Geometry check sheet. Reference: the model listing, model coordinates, mm. Face numbers are marked on the shaded views. A direction names the side the tool comes from. Give positions to 0.01 mm unless a question says otherwise; leave off trailing zeros. Write each loop counter-clockwise with the first axis right and the second up, starting at its lowest first coordinate (ties: lowest second). Pieces come first, ordered by that corner, then holes.
(1) Cross-section at C-C (z = -8). Record the boundary of the cut face in (x, y), and give its area (3 significant figures).
(2) Cross-section at B-B (y = 13.25). Record the boundary of the cut face in (x, z).
(3) Cross-section at A-A (z = 3). Record the boundary of the cut face in (x, y).
(4) Tool access check on the marked faces 4, 5, 6 and 7. Record the directions out of +Z, -Z, +X, -X, +Y, -Y that give a thin tool (end or side, any length) a straight path to the whole face; none if there is none.
(5) Mould release check, pull along Z, two halves, no side actions. Record for the marked faces 1, 2 and 3: +Z half, -Z half, draft (parallel to the pull), parting line (faces both ways), or undercut.
(6) Thickness scan on line 1 along Z through (x, y) = (-8.75, 5); line 2 along X through (y, z) = (10, -0.5); line 3 along Y through (x, z) = (22, 3.65). Record the ranges inside material, lowest first.
(7) Cross-section at D-D (x = 15). Record the boundary of the cut face in (y, z), and give its area (3 significant figures).
(8) Depth check by flat-ended pin: P1, Ø5, axis at x = -9, y = 8, coming from the -Z side; P2, Ø5, axis at x = 13.5, z = -1.5, coming from the -Y side; P3, Ø3, axis at x = 22, y = 9.5, coming from the -Z side; P4, Ø8, axis at x = 13.5, y = 13, coming from the +Z side. Enter the tip coordinate at first touch or a pass-through.
```python
from build123d import *

# Parameters (mm, degrees)
SKETCH1_W           = 50
SKETCH1_H           = 36
BOSS_EXTRUDE1_DEPTH = 3
SKETCH2_W           = 5
SKETCH2_H           = 8
SKETCH2_W_2         = 6
SKETCH2_H_2         = 20
BOSS_EXTRUDE2_DEPTH = 14
SKETCH3_W           = 15
SKETCH3_H           = 4
BOSS_EXTRUDE3_DEPTH = 13
SKETCH4_R           = 3
BOSS_EXTRUDE4_DEPTH = 2
SKETCH5_R           = 2
CUT_EXTRUDE1_DEPTH  = 12
CUT_EXTRUDE2_DEPTH  = 11
SKETCH7_W           = 1.666666666
SKETCH7_H           = 10
BOSS_EXTRUDE5_DEPTH = 14
CUT_EXTRUDE3_REACH  = 45.218
CUT_EXTRUDE4_REACH  = 36.943
SKETCH10_W          = 10
SKETCH10_H          = 1.666666667
BOSS_EXTRUDE7_DEPTH = 13
CUT_EXTRUDE5_DEPTH  = 2
SKETCH12_R          = 2
CUT_EXTRUDE6_DEPTH  = 6
CHAMFER1_SIZE       = 2
CHAMFER1_SIZE2      = 4
CUT_EXTRUDE7_DEPTH  = 5
SKETCH14_R          = 1.3
CUT_EXTRUDE8_DEPTH  = 6
SKETCH15_R          = 1
CUT_EXTRUDE9_DEPTH  = 6


with BuildPart() as part:
    # Sketch1 → Boss-Extrude1 (new body)
    with BuildSketch(Plane(origin=(0, 0, 0), x_dir=(1, 0, 0), z_dir=(0, 1, 0))):
        Rectangle(SKETCH1_W, SKETCH1_H)
    extrude(amount=BOSS_EXTRUDE1_DEPTH)

    # Sketch2 → Boss-Extrude2 (add)
    with BuildSketch(Plane(origin=(0, 3, 0), x_dir=(1, 0, 0), z_dir=(0, 1, 0))):
        with Locations((22.5, -4)):
            Rectangle(SKETCH2_W, SKETCH2_H)
        with Locations((-8, 2)):
            Rectangle(SKETCH2_W_2, SKETCH2_H_2)
    extrude(amount=BOSS_EXTRUDE2_DEPTH)

    # Sketch3 → Boss-Extrude3 (add)
    with BuildSketch(Plane(origin=(0, 3, 0), x_dir=(1, 0, 0), z_dir=(0, 1, 0))):
        with Locations((10, 16)):
            Rectangle(SKETCH3_W, SKETCH3_H)
    extrude(amount=BOSS_EXTRUDE3_DEPTH)

    # Sketch4 → Boss-Extrude4 (add)
    with BuildSketch(Plane(origin=(0, 0, -18), x_dir=(-1, 0, 0), z_dir=(0, 0, -1))):
        with Locations(Location((-13.5, 9.25, 0), (0, 0, 180))):
            Circle(SKETCH4_R)
    extrude(amount=BOSS_EXTRUDE4_DEPTH)

    # Sketch5 → Cut-Extrude1 (cut)
    with BuildSketch(Plane(origin=(0, 0, -20), x_dir=(-1, 0, 0), z_dir=(0, 0, -1))):
        with Locations((-13.5, 9.25)):
            Circle(SKETCH5_R)
    extrude(amount=-CUT_EXTRUDE1_DEPTH, mode=Mode.SUBTRACT)

    # Sketch6 → Cut-Extrude2 (cut)
    with BuildSketch(Plane(origin=(0, 3, 0), x_dir=(1, 0, 0), z_dir=(0, 1, 0))):
        Polygon((-11, 12), (-11, 18), (-25, 18), (-25, -18), (25, -18), (25, -8), (-11, -8), align=None)
    extrude(amount=-CUT_EXTRUDE2_DEPTH, mode=Mode.SUBTRACT)

    # Sketch7 → Boss-Extrude5 (add)
    with BuildSketch(Plane(origin=(0, 17, 0), x_dir=(1, 0, 0), z_dir=(0, 1, 0))):
        with Locations((22.5, 5)):
            Rectangle(SKETCH7_W, SKETCH7_H)
    extrude(amount=-BOSS_EXTRUDE5_DEPTH)

    # Sketch8 → Cut-Extrude3 (cut, up to next)
    with BuildSketch(Plane(origin=(23.333333333, 0, 0), x_dir=(0, 0, -1), z_dir=(1, 0, 0)), mode=Mode.PRIVATE) as cut_extrude3_sk1:
        Polygon((10, 3), (0, 17), (10, 17), align=None)
    cut_extrude3_tool1 = extrude(cut_extrude3_sk1.sketch, amount=-CUT_EXTRUDE3_REACH, mode=Mode.PRIVATE) & part.part
    add(cut_extrude3_tool1.solids().sort_by_distance((23.333333, 12.333333, -6.666667))[0], mode=Mode.SUBTRACT)

    # Sketch9 → Cut-Extrude4 (cut, up to next)
    with BuildSketch(Plane(origin=(0, 3, 0), x_dir=(1, 0, 0), z_dir=(0, 1, 0)), mode=Mode.PRIVATE) as cut_extrude4_sk1:
        Polygon((25, 0), (23.333333333, 0), (23.333333333, 10), (17.5, 18), (25, 18), align=None)
    cut_extrude4_tool1 = extrude(cut_extrude4_sk1.sketch, amount=-CUT_EXTRUDE4_REACH, mode=Mode.PRIVATE) & part.part
    add(cut_extrude4_tool1.solids().sort_by_distance((22.951389, 3, -11.770833))[0], mode=Mode.SUBTRACT)

    # Sketch10 → Boss-Extrude7 (add)
    with BuildSketch(Plane(origin=(0, 3, 0), x_dir=(1, 0, 0), z_dir=(0, 1, 0))):
        with Locations((-2.5, 15.666666666)):
            Rectangle(SKETCH10_W, SKETCH10_H)
    extrude(amount=BOSS_EXTRUDE7_DEPTH)

    # Sketch11 → Cut-Extrude5 (cut)
    with BuildSketch(Plane(origin=(0, 0, -16.5), x_dir=(-1, 0, 0), z_dir=(0, 0, -1))):
        Polygon((7.5, 3), (-2.5, 16), (7.5, 16), align=None)
    extrude(amount=-CUT_EXTRUDE5_DEPTH, mode=Mode.SUBTRACT)

    # Sketch12 → Cut-Extrude6 (cut)
    with BuildSketch(Plane.ZY.offset(11)):
        with Locations((4, 5)):
            Circle(SKETCH12_R)
        with Locations((-8, 12)):
            Circle(SKETCH12_R)
    extrude(amount=-CUT_EXTRUDE6_DEPTH, mode=Mode.SUBTRACT)

    # Chamfer1
    chamfer1_edges = [part.edges().sort_by_distance(p)[0] for p in [
        (10, 3, -14),
    ]]
    chamfer1_side = [part.faces().sort_by_distance(p)[0] for p in [
        (7.078272128, 3, -4.239053672),
    ]]
    chamfer(chamfer1_edges, length=CHAMFER1_SIZE, length2=CHAMFER1_SIZE2, reference=chamfer1_side[0])

    # Sketch13 → Cut-Extrude7 (cut)
    with BuildSketch(Plane(origin=(0, 3, 0), x_dir=(1, 0, 0), z_dir=(0, 1, 0))):
        Polygon((-7.5, 16.5), (-11, 12), (-11, 18), (2.5, 18), (2.5, 16.5), align=None)
    extrude(amount=-CUT_EXTRUDE7_DEPTH, mode=Mode.SUBTRACT)

    # Sketch14 → Cut-Extrude8 (cut)
    with BuildSketch(Plane(origin=(0, 17, 0), x_dir=(1, 0, 0), z_dir=(0, 1, 0))):
        with Locations(Location((6.5, 16, 0), (0, 0, 270))):
            Circle(SKETCH14_R)
        with Locations(Location((-8, 2, 0), (0, 0, 270))):
            Circle(SKETCH14_R)
        with Locations(Location((22.5, -3, 0), (0, 0, 270))):
            Circle(SKETCH14_R)
    extrude(amount=-CUT_EXTRUDE8_DEPTH, mode=Mode.SUBTRACT)

    # Sketch15 → Cut-Extrude9 (cut)
    with BuildSketch(Plane.XY.offset(8)):
        with Locations((-7, 9.5)):
            Circle(SKETCH15_R)
        with Locations((22, 9.5)):
            Circle(SKETCH15_R)
    extrude(amount=-CUT_EXTRUDE9_DEPTH, mode=Mode.SUBTRACT)


solid = part.part
```
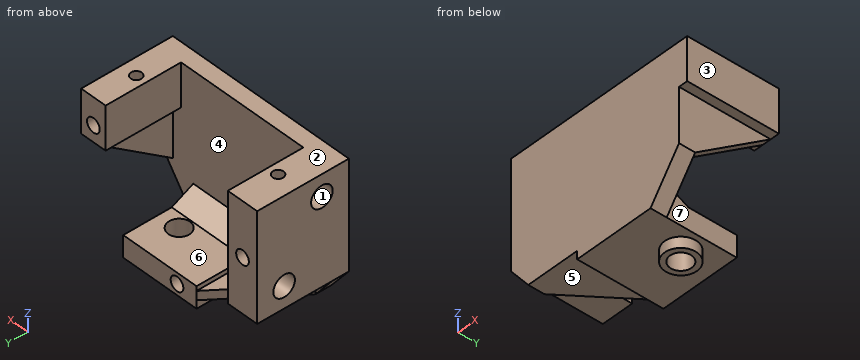
Reply:
1. outline: (-11, 0) - (23.33, 0) - (23.33, 5.8) - (21.67, 5.8) - (21.67, 3) - (-5, 3) - (-5, 10) - (-11, 10) - close; (-11, 14) - (-5, 14) - (-5, 17) - (-11, 17) - close
1. area: 168 mm2
2. outline: (-11, -12) - (-5, -12) - (-5, -9.56) - (-11, -9.56) - close; (-11, -6.44) - (-5, -6.44) - (-5, 8) - (-11, 8) - close; (0.38, -16.5) - (2.5, -16.5) - (2.5, -18) - (17.5, -18) - (17.5, -14) - (2.5, -14) - (2.5, -14.83) - (0.38, -14.83) - close; (20, 0) - (21.67, 0) - (21.67, -2.68) - (23.33, -2.68) - (23.33, 0) - (25, 0) - (25, 8) - (20, 8) - close; hole circle Ø2.6 at (-8, -2); hole circle Ø2.6 at (6.5, -16); hole circle Ø2.6 at (22.5, 3)
3. outline: (-11, 0) - (25, 0) - (25, 17) - (23.8, 17) - (23.8, 11) - (21.2, 11) - (21.2, 17) - (20, 17) - (20, 3) - (-5, 3) - (-5, 3.27) - (-11, 3.27) - close; (-11, 6.73) - (-5, 6.73) - (-5, 17) - (-11, 17) - close; hole circle Ø2 at (-7, 9.5); hole circle Ø2 at (22, 9.5)
4. face 4: +Y
4. face 5: -Z, -X, +Y, -Y
4. face 6: +Z, +X, -X, +Y
4. face 7: +Z, -Z, +X, +Y
5. face 1: undercut
5. face 2: +Z half
5. face 3: draft
6. line 1: z = -12 to 2, 6 to 8
6. line 2: x = -11 to -5, 21.67 to 23.33
6. line 3: y = 0 to 8.5, 10.5 to 11
7. outline: (0, -18) - (6.65, -18) - (6.65, -20) - (7.93, -20) - (7.93, -14) - (7, -14) - (3, -12) - (3, 8) - (0, 8) - close; (10.57, -20) - (11.85, -20) - (11.85, -18) - (16, -18) - (16, -14) - (10.57, -14) - close
7. area: 129 mm2
8. P1: stops at z = -12
8. P2: stops at y = 0
8. P3: stops at z = -6.43
8. P4: stops at z = -14
